```python
from build123d import *

# Parameters (mm, degrees)
F1_DEPTH = 38.1
F2_W     = 58.2091789693
F2_H     = 15.3594079479
F3_DEPTH = 76.2
F5_DEPTH = 50.8
F6_W     = 76.010748744
F6_H     = 27.6595102623
F7_DEPTH = 7.62
F8_R     = 7.6303567528
F8_R_2   = 7.7116101736
F8_R_3   = 7.8878838381
F9_DEPTH = 38.1


with BuildPart() as f1:
    # F0 (on Front) → F1 (new body, symmetric)
    with BuildSketch(Plane.XZ):
        Polygon((-76.010748744, 63.9190971851), (-76.010748744, 0), (0, 0), (76.4603540301, 0), (0, 63.9190971851), align=None)
    extrude(amount=F1_DEPTH, both=True)

    # F2 (on face) → F3 (cut, symmetric)
    with BuildSketch(Plane.XZ.offset(38.1)):
        with Locations((-46.9061592594, 7.679703974)):
            Rectangle(F2_W, F2_H)
    extrude(amount=F3_DEPTH, both=True, mode=Mode.SUBTRACT)

    # F4 (on Top) → F5 (cut, symmetric)
    with BuildSketch(Plane.XY):
        Polygon((19.974257797, -22.5624050945), (19.974257797, -38.3158996701), (76.5146613121, -38.1380990148), (76.5146613121, -22.5624050945), align=None)
    extrude(amount=F5_DEPTH, both=True, mode=Mode.SUBTRACT)

    # F6 (on face) → F7 (cut)
    with BuildSketch(Plane.XY.offset(63.9190971851)):
        with Locations((-38.005374372, 0.5322289653)):
            Rectangle(F6_W, F6_H)
        Polygon((0, 14.3619840965), (0, -13.2975261658), (15.1856476441, -13.2975261658), (15.1856476441, 14.5155396312), align=None)
    extrude(amount=-F7_DEPTH, mode=Mode.SUBTRACT)

    # F8 (on face) → F9 (cut, symmetric)
    with BuildSketch(Plane(origin=(31.4534289532, 0, 37.6247540897), x_dir=(0.7672228325, 0, -0.6413806399), z_dir=(0.6413806399, 0, 0.7672228325))):
        with Locations((0, -8.2661788911)):
            Circle(F8_R)
        with Locations((32.8613109887, -8.2661788911)):
            Circle(F8_R_2)
        with Locations((0, 24.0339674056)):
            Circle(F8_R)
        with Locations((32.8613109887, 24.0339674056)):
            Circle(F8_R_3)
    extrude(amount=F9_DEPTH, both=True, mode=Mode.SUBTRACT)


solid = f1.part
```
Geometry: final body of the model. Coordinates: model frame, mm. A direction names the side the tool comes from. Give positions to 0.01 mm unless a question says otherwise; leave off trailing zeros. Order: outer loops, then holes, each group sorted by start corner. A loop starts at its lowest first (then second) coordinate and runs counter-clockwise, first axis right, second up. Notation, with made-up numbers: M 69,-31.75 L 83,-31.75 A20 cw 83,7.25 Z; hole C 70,81.25 d8. An arc over 180 degrees is marked long. Answer as CSV lines item,"result". Start each with the question number.
1) Cut plane B-B (y = -5). Output: boundary loops of the cut face in (x, z).
2) Set-up query: faces 4 (the flat face through (19.974, -30, 24)), 5 (the flat face through (-34, -13.298, 60)), 6 (the flat face through (-17.802, -1, 8)). Return all of +Z, -Z, +X, -X, +Y, -Y with unobstructed straight access to the full face (end or side cutting, diameter ignored); none if empty.
3) Cut plane D-D (y = 19). Output: boundary loops of the cut face in (x, z), then the cut area to 3 significant figures.
4) Cut plane A-A (y = -30). Output: boundary loops of the cut face in (x, z), then the cut area to 3 significant figures.
5) Cut plane C-C (x = -40). Output: boundary loops of the cut face in (y, z), then the cut area to 3 significant figures.
6) Mould query, pull axis Z, two halves, no side actions, for faces 1 (the cylindrical face through (18.64, 31.6, 23.85)), 2 (the flat face through (29, -1, 0)), 3 (the flat face through (-34, 1, 56.299)). Classes: +Z half, -Z half, draft (parallel to the pull), parting line (faces both ways), or undercut.
7) First-contact query: P1, Ø4, axis at x = 25, y = 23, coming from the +Z side; P2, Ø1, axis at x = 45.5, z = 9, coming from the -Y side; P3, Ø4.5, axis at y = -28, z = 19, coming from the +X side. Flat tips, straight axial feed; report the tip coordinate or a pass-through.
8) Line query: line 1 (Y direction, x = 11.5, z = 22); line 2 (Z direction, x = -65.5, y = -4); line 3 (Y direction, x = -63, z = 57). Output: solid intervals per line, ascending. Write a range as from..to.
Findings below:
1,outline,"M -76.01,15.36 L -17.8,15.36 L -17.8,0 L 33.73,0 L 51.31,21.03 L 36.74,33.2 L 12.31,3.97 L 1.73,12.82 L 26.16,42.05 L 9.12,56.3 L -76.01,56.3 Z; M 51.94,0 L 76.46,0 L 62.03,12.07 Z"
2,face 4,"+Z, -Z, +X, -Y"
2,face 5,"+Z, +X, -X"
2,face 6,"-Z, -X, +Y, -Y"
3,outline,"M -76.01,15.36 L -17.8,15.36 L -17.8,0 L 34.92,0 L 52.01,20.44 L 35.85,33.95 L 11.42,4.72 L 2.62,12.07 L 27.05,41.3 L 0,63.92 L -76.01,63.92 Z; M 50.75,0 L 76.46,0 L 61.32,12.65 Z"
3,area,"5,710 mm²"
4,outline,"M -76.01,15.36 L -17.8,15.36 L -17.8,0 L 19.97,0 L 19.97,47.22 L 0,63.92 L -76.01,63.92 Z"
4,area,"5,070 mm²"
5,outline,"M -38.1,15.36 L 38.1,15.36 L 38.1,63.92 L 14.36,63.92 L 14.36,56.3 L -13.3,56.3 L -13.3,63.92 L -38.1,63.92 Z"
5,area,"3,490 mm²"
6,face 1,"undercut"
6,face 2,"-Z half"
6,face 3,"+Z half"
7,P1,"stops at z = 44.69"
7,P2,"stops at y = -22.56"
7,P3,"stops at x = 19.97"
8,line 1,"y = -38.1..-13.77, -2.76..18.53, 29.54..38.1"
8,line 2,"z = 15.36..56.3"
8,line 3,"y = -38.1..-13.3, 14.36..38.1"
